from build123d import *

# Parameters (mm, degrees)
SKETCH_1_W          = 110.7
SKETCH_1_H          = 38.85
EXTRUDE_1_DEPTH     = 1
SKETCH_2_W          = 33.45
SKETCH_2_H          = 105.3
EXTRUDE_2_DEPTH     = 0.5
SKETCH_3_W          = 22.339400882
SKETCH_3_H          = 24.25
CUT_EXTRUDE_1_DEPTH = 2


with BuildPart() as part:
    # Эскиз1 → Бобышка-Вытянуть1 (new body)
    with BuildSketch(Plane(origin=(0.5, 0, 0), x_dir=(0, -1, 0), z_dir=(0, 0, 1))):
        with Locations((-45.5, 22.825)):
            Rectangle(SKETCH_1_W, SKETCH_1_H)
    extrude(amount=-EXTRUDE_1_DEPTH)

    # Эскиз2 → Бобышка-Вытянуть2 (add)
    with BuildSketch(Plane.XY):
        with Locations((22.825, 45.5)):
            Rectangle(SKETCH_2_W, SKETCH_2_H)
    extrude(amount=EXTRUDE_2_DEPTH)

    # Эскиз3 → Вырез-Вытянуть1 (cut)
    with BuildSketch(Plane.XY.offset(0.5)):
        with Locations((17.385892666, 42.275)):
            Rectangle(SKETCH_3_W, SKETCH_3_H)
        with Locations((17.385892666, 9.819443695)):
            Rectangle(SKETCH_3_W, SKETCH_3_H)
    extrude(amount=-CUT_EXTRUDE_1_DEPTH, mode=Mode.SUBTRACT)


solid = part.part
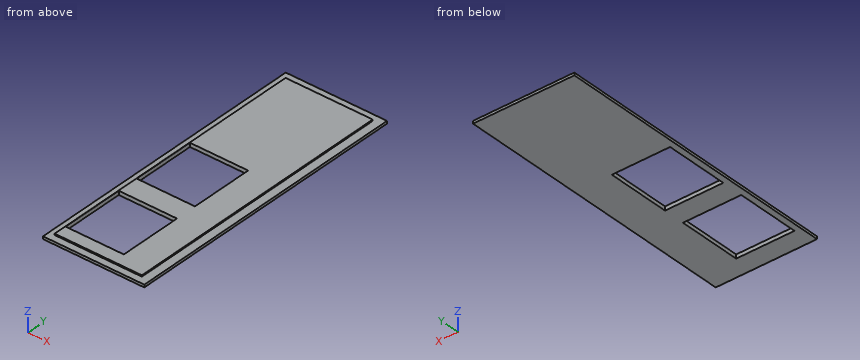
The listing builds one solid part. Answer for the finished solid, in the listing's coordinates (mm). Coordinates: 2 decimals unless noted, no trailing zeros. Write each loop counter-clockwise with the first axis right and the second up, starting at its lowest first coordinate (ties: lowest second). Pieces come first, ordered by that corner, then holes. Notation, with made-up numbers: (-34.75, -2) - (17.25, -2) arc R27 cw to (17.25, 27) - close; hole circle Ø3 at (-5, -13.75). An arc over 180 degrees is marked (long way). Return JSON: item names as keys, results as strings.
1. Consider line 1 along Y through (x, z) = (28, -0.3); line 2 along Y through (x, z) = (17, 0.1); line 3 along X through (y, z) = (36.5, -0.85). Determine where each line is inside the solid, lowest interval first.
Final values:
{"line 1": "-9.85 to -2.31, 21.94 to 30.15, 54.4 to 100.85", "line 2": "-7.15 to -2.31, 21.94 to 30.15, 54.4 to 98.15", "line 3": "3.9 to 6.22, 28.56 to 42.75"}
2. The part is cut by section B-B on z = 0.25. Determine the outline of the cut face in (x, y).
Final values:
{"outline": "(6.1, -7.15) - (39.55, -7.15) - (39.55, 98.15) - (6.1, 98.15) - close; hole (6.22, -2.31) - (28.56, -2.31) - (28.56, 21.94) - (6.22, 21.94) - close; hole (6.22, 30.15) - (28.56, 30.15) - (28.56, 54.4) - (6.22, 54.4) - close"}
3. The part is cut by section C-C on y = 11. Determine the outline of the cut face in (x, z), then the cut area to 3 significant figures.
Final values:
{"outline": "(3.9, -1) - (6.22, -1) - (6.22, 0.5) - (6.1, 0.5) - (6.1, 0) - (3.9, 0) - close; (28.56, -1) - (42.75, -1) - (42.75, 0) - (39.55, 0) - (39.55, 0.5) - (28.56, 0.5) - close", "area": "22.1 mm^2"}
4. The part is cut by section D-D on y = 61. Determine the outline of the cut face in (x, z).
Final values:
{"outline": "(3.9, -1) - (42.75, -1) - (42.75, 0) - (39.55, 0) - (39.55, 0.5) - (6.1, 0.5) - (6.1, 0) - (3.9, 0) - close"}
5. The part is cut by section A-A on x = 15. Determine the outline of the cut face in (y, z).
Final values:
{"outline": "(-9.85, -1) - (-2.31, -1) - (-2.31, 0.5) - (-7.15, 0.5) - (-7.15, 0) - (-9.85, 0) - close; (21.94, -1) - (30.15, -1) - (30.15, 0.5) - (21.94, 0.5) - close; (54.4, -1) - (100.85, -1) - (100.85, 0) - (98.15, 0) - (98.15, 0.5) - (54.4, 0.5) - close"}
6. This flat-tipped pin is pushed along its axis until it touches: pin 1 Ø0.6 at (x, z) = (23, 0.5) entering from +Y. Where does it stop, or does it pass through?
Final values:
{"pin 1": "y = 98.15"}
